from build123d import *

# Parameters (mm, degrees)
F0_W     = 40
F0_H     = 40
F1_DEPTH = 3
F2_W     = 8
F2_H     = 3
F2_W_2   = 3
F2_H_2   = 8
F3_DEPTH = 3.001
F4_W     = 8.44
F4_H     = 3.22
F4_W_2   = 8
F4_H_2   = 0.22
F4_W_3   = 0.22
F4_H_3   = 8
F5_DEPTH = 3.001


with BuildPart() as f1:
    # F0 (on Top) → F1 (new body)
    with BuildSketch(Plane.XY):
        Rectangle(F0_W, F0_H)
    extrude(amount=F1_DEPTH)

    # F2 (on face) → F3 (cut, through all)
    with BuildSketch(Plane(origin=(0, 0, 0), x_dir=(1, 0, 0), z_dir=(0, 0, -1))):
        with Locations((-8, -18.5)):
            Rectangle(F2_W, F2_H)
        with Locations((8, -18.5)):
            Rectangle(F2_W, F2_H)
        with Locations((16, 18.5)):
            Rectangle(F2_W, F2_H)
        with Locations((0, 18.5)):
            Rectangle(F2_W, F2_H)
        with Locations((-18.5, -8)):
            Rectangle(F2_W_2, F2_H_2)
        with Locations((-18.5, 8)):
            Rectangle(F2_W_2, F2_H_2)
        with Locations((18.5, -8)):
            Rectangle(F2_W_2, F2_H_2)
        with Locations((18.5, 8)):
            Rectangle(F2_W_2, F2_H_2)
        with Locations((-16, 18.5)):
            Rectangle(F2_W, F2_H)
    extrude(amount=-F3_DEPTH, mode=Mode.SUBTRACT)

    # F4 (on face) → F5 (cut, through all)
    with BuildSketch(Plane(origin=(0, 0, 0), x_dir=(1, 0, 0), z_dir=(0, 0, -1))):
        with Locations((-8, -18.39)):
            Rectangle(F4_W, F4_H)
        with Locations((8, -18.39)):
            Rectangle(F4_W, F4_H)
        with Locations((-16, 16.89)):
            Rectangle(F4_W_2, F4_H_2)
        with Locations((0, 16.89)):
            Rectangle(F4_W_2, F4_H_2)
        with Locations((16, 16.89)):
            Rectangle(F4_W_2, F4_H_2)
        with Locations((-16.89, -8)):
            Rectangle(F4_W_3, F4_H_3)
        with Locations((-16.89, 8)):
            Rectangle(F4_W_3, F4_H_3)
        with Locations((16.89, -8)):
            Rectangle(F4_W_3, F4_H_3)
        with Locations((16.89, 8)):
            Rectangle(F4_W_3, F4_H_3)
    extrude(amount=-F5_DEPTH, mode=Mode.SUBTRACT)


solid = f1.part
Input: part model. Units: mm. Frame: model coordinates. A direction names the side the tool comes from. Round coordinates to 2 decimals unless told otherwise and drop trailing zeros. Order: outer loops, then holes, each group sorted by start corner. A loop starts at its lowest first (then second) coordinate and runs counter-clockwise, first axis right, second up. Notation, with made-up numbers: (-34, 44.5) - (-7, 44.5) arc R19 ccw to (-7, 77.5) - close; hole circle Ø2 at (-23.75, 67). An arc over 180 degrees is marked (long way). Use a Markdown table: item, result.
1. First-contact query: pin 1 (1.5 mm diameter, centred on x = -9.5, z = 1, fed in from +Y); pin 2 (0.9 mm diameter, centred on x = 1.5, z = 1.5, fed in from -Y); pin 3 (0.9 mm diameter, centred on y = -18, z = 2, fed in from -X). Flat tips, straight axial feed; report the tip coordinate or a pass-through.
Evaluation:
| item | result |
|---|---|
| pin 1 | y = 16.78 |
| pin 2 | y = -16.78 |
| pin 3 | x = -12 |
2. Material intervals for probe 1 along Y at (x, z) = (18, 1); probe 2 along X at (y, z) = (18, 0.3); probe 3 along X at (y, z) = (-17, 1.7), sorted ascending.
Evaluation:
| item | result |
|---|---|
| probe 1 | -16.78 to -12, -4 to 4, 12 to 20 |
| probe 2 | -20 to -12.22, -3.78 to 3.78, 12.22 to 20 |
| probe 3 | -12 to -4, 4 to 12 |
3. Access query for faces 1 (the face through (-8, 16.78, 1)), 2 (the face through (16, -16.78, 1)), 3 (the face through (4, -18, 1)), 4 (the face through (18, -12, 1)). Directions: +Z, -Z, +X, -X, +Y, -Y. A direction counts if a zero-diameter tool reaches every point of the face in a straight line with its end or side. Return the directions, or none.
Evaluation:
| item | result |
|---|---|
| face 1 | +Z, -Z, +Y |
| face 2 | +Z, -Z, +X, -Y |
| face 3 | +Z, -Z, -Y |
| face 4 | +Z, -Z, +X |
4. Mould query, pull axis Y, two halves, no side actions, for faces 5 (the face through (0, 20, 1)), 6 (the face through (-16.78, 8, 1)), 7 (the face through (20, -14, 1)), 8 (the face through (-18, -4, 1)). Classes: +Y half, -Y half, draft (parallel to the pull), parting line (faces both ways), or undercut.
Evaluation:
| item | result |
|---|---|
| face 5 | +Y half |
| face 6 | undercut |
| face 7 | draft |
| face 8 | undercut |
5. Section A-A on y = 5. Return the cut outline in (x, z), then the cut area to 3 significant figures.
Evaluation:
| item | result |
|---|---|
| outline | (-16.78, 0) - (16.78, 0) - (16.78, 3) - (-16.78, 3) - close |
| area | 101 mm^2 |
6. Section B-B on x = -8.5. Return the cut outline in (y, z), then the cut area to 3 significant figures.
Evaluation:
| item | result |
|---|---|
| outline | (-20, 0) - (16.78, 0) - (16.78, 3) - (-20, 3) - close |
| area | 110 mm^2 |
